Read the model definition and answer for the solid it produces. Units are mm, in the model's axes. A direction names the side the tool comes from. Give positions to 0.01 mm unless a question says otherwise; leave off trailing zeros. Order: outer loops, then holes, each group sorted by start corner. A loop starts at its lowest first (then second) coordinate and runs counter-clockwise, first axis right, second up. Notation, with made-up numbers: (0.5, -31) - (51.5, -31) arc R19 cw to (51.5, 6) - close; hole circle Ø1 at (68, 16). An arc over 180 degrees is marked (long way). One line per item, written item: value. Start each with the question number.
```python
from build123d import *

# Parameters (mm, degrees)
BOSS_EXTRUDE1_DEPTH   = 102.108
SKETCH2_W             = 76.708
SKETCH2_H             = 76.2
CUT_EXTRUDE1_DEPTH    = 220.104116036
F_7_0MM_DOWEL_HOLE1_D = 7
FILLET1_R             = 6.35
SKETCH5_R             = 2.38125
CUT_EXTRUDE2_DEPTH    = 220.104116036


with BuildPart() as part:
    # Sketch1 → Boss-Extrude1 (new body)
    with BuildSketch(Plane(origin=(0, 0, 0), x_dir=(0, 0, -1), z_dir=(1, 0, 0))):
        Polygon((0, 0), (-165.1, 0), (-165.1, 50.8), (-25.4, 50.8), (-25.4, 101.6), (0, 101.6), align=None)
    extrude(amount=BOSS_EXTRUDE1_DEPTH)

    # Sketch2 → Cut-Extrude1 (cut, through all)
    with BuildSketch(Plane(origin=(0, 0, 0), x_dir=(-1, 0, 0), z_dir=(0, 0, -1))):
        with Locations((-51.054, 38.1)):
            Rectangle(SKETCH2_W, SKETCH2_H)
    extrude(amount=-CUT_EXTRUDE1_DEPTH, mode=Mode.SUBTRACT)

    # Ø7.0mm Dowel Hole1 (through all)
    with Locations(Plane(origin=(0, 101.6, 0), x_dir=(1, 0, 0), z_dir=(0, 1, 0))):
        with Locations((50.8, -12.7)):
            Hole(F_7_0MM_DOWEL_HOLE1_D / 2)

    # Fillet1
    fillet1_edges = [part.edges().sort_by_distance(p)[0] for p in [
        (95.758, 50.8, 25.4),
        (6.35, 50.8, 25.4),
        (89.408, 76.2, 12.7),
        (12.7, 76.2, 12.7),
        (0, 101.6, 12.7),
        (102.108, 101.6, 12.7),
    ]]
    fillet(fillet1_edges, radius=FILLET1_R)

    # Sketch5 → Cut-Extrude2 (cut, through all)
    with BuildSketch(Plane(origin=(102.108, 0, 0), x_dir=(0, 0, -1), z_dir=(1, 0, 0))):
        with Locations((-146.05, 25.4)):
            Circle(SKETCH5_R)
        with Locations((-88.9, 25.4)):
            Circle(SKETCH5_R)
        with Locations((-69.85, 25.4)):
            Circle(SKETCH5_R)
    extrude(amount=-CUT_EXTRUDE2_DEPTH, mode=Mode.SUBTRACT)


solid = part.part
```
1) The mould has two halves that part along Z. Classify faces 1 (the flat face through (6, 25, 165.1)), 2 (the flat face through (52, 76.2, 18)), 3 (the cylindrical face through (6.44, 26.12, 86.63)): +Z half, -Z half, draft (parallel to the pull), parting line (faces both ways), or undercut.
2) Section D-D on z = 146.05 is taken. Write down the section's boundary in (x, y), plus the area to 3 significant figures.
3) For faces 4 (the cylindrical face through (95.85, 52.71, 27.21)), 5 (the flat face through (89.408, 27, 81)), determine the directions among +Z, -Z, +X, -X, +Y, -Y from which every point of the face is accessible in a straight line to the end or side of a thin tool.
4) Section A-A on y = 25.4 is taken. Give the number of separate pieces and of enclosed holes in the cut face, plus the area to 3 significant figures.
5) Each of these flat-tipped pins is pushed along its axis until it touches: pin 1 (14 mm diameter, centred on x = 3.5, z = 81.5, fed in from +Y); pin 2 (7.5 mm diameter, centred on x = 55.5, z = 16, fed in from -Y). Where does it stop, or does it pass through?
6) Section B-B on y = 61.5 is taken. Write down the section's boundary in (x, z).
7) Find the intervals of material crossed by probe 1 along Z at (x, y) = (7, 25); probe 2 along X at (y, z) = (41, 135); probe 3 along Y at (x, z) = (96.25, 146.05), in increasing order. Write a range as from..to.
8) Section C-C on x = 50.8 is taken. Write down the section's boundary in (y, z).
Solved:
1. face 1: +Z half
1. face 2: draft
1. face 3: undercut
2. outline: (0, 0) - (12.7, 0) - (12.7, 23.02) - (0, 23.02) - close; (0, 27.78) - (12.7, 27.78) - (12.7, 50.8) - (0, 50.8) - close; (89.41, 0) - (102.11, 0) - (102.11, 23.02) - (89.41, 23.02) - close; (89.41, 27.78) - (102.11, 27.78) - (102.11, 50.8) - (89.41, 50.8) - close
2. area: 1,170 mm2
3. face 4: +Z, +X, -X, +Y
3. face 5: +Z, -Z, -Y
4. separate pieces: 8
4. enclosed holes: 0
4. area: 3,830 mm2
5. pin 1: stops at y = 50.8
5. pin 2: stops at y = 76.2
6. outline: (0, 0) - (12.7, 0) - (12.7, 25.4) - (0, 25.4) - close; (89.41, 0) - (102.11, 0) - (102.11, 25.4) - (89.41, 25.4) - close
7. probe 1: z = 0..67.5, 72.2..86.55, 91.25..143.7, 148.4..165.1
7. probe 2: x = 0..12.7, 89.41..102.11
7. probe 3: y = 0..23.02, 27.78..50.8
8. outline: (76.2, 0) - (101.6, 0) - (101.6, 9.2) - (76.2, 9.2) - close; (76.2, 16.2) - (101.6, 16.2) - (101.6, 25.4) - (76.2, 25.4) - close
